from build123d import *

# Parameters (mm, degrees)
SKETCH1_W           = 297.73626
SKETCH1_H           = 182.7784
BOSS_EXTRUDE1_DEPTH = 15.24
CUT_EXTRUDE1_DEPTH  = 350.695698609
CUT_EXTRUDE2_DEPTH  = 350.695698609
SKETCH5_W           = 297.73626
SKETCH5_H           = 50.702926555
BOSS_EXTRUDE2_DEPTH = 76.2
FILLET1_R           = 12.7
FILLET2_R           = 12.7
SKETCH6_R           = 16.245750799
BOSS_EXTRUDE3_DEPTH = 50.8
SKETCH7_R           = 11.813796097
BOSS_EXTRUDE4_DEPTH = 12.7
CHAMFER1_SIZE       = 10
SKETCH8_R           = 1.248823532
CUT_EXTRUDE3_DEPTH  = 12.7
BOSS_EXTRUDE5_DEPTH = 12.7
BOSS_EXTRUDE6_DEPTH = 89.408
SKETCH11_W          = 104.0892
SKETCH11_H          = 178.532208179
BOSS_EXTRUDE7_DEPTH = 3.048
SKETCH12_R          = 15.475849778
SKETCH12_R_2        = 18.114114382
SKETCH12_R_3        = 14.983279797
BOSS_EXTRUDE8_DEPTH = 12.192


with BuildPart() as part:
    # Sketch1 → Boss-Extrude1 (new body)
    with BuildSketch(Plane(origin=(0, 0, 0), x_dir=(1, 0, 0), z_dir=(0, 1, 0))):
        with Locations((148.86813, 91.3892)):
            Rectangle(SKETCH1_W, SKETCH1_H)
    extrude(amount=BOSS_EXTRUDE1_DEPTH)

    # Sketch2 → Cut-Extrude1 (cut, through all)
    with BuildSketch(Plane.ZY):
        with BuildLine():
            ThreePointArc((-43.45432, 0), (-56.15432, 12.7), (-68.85432, 0))
            Line((-68.85432, 0), (-43.45432, 0))
        make_face()
        with BuildLine():
            ThreePointArc((-113.92408, 0), (-126.62408, 12.7), (-139.32408, 0))
            Line((-139.32408, 0), (-126.62408, 0))
            Line((-126.62408, 0), (-113.92408, 0))
        make_face()
    extrude(amount=-CUT_EXTRUDE1_DEPTH, mode=Mode.SUBTRACT)

    # Sketch4 → Cut-Extrude2 (cut, through all)
    with BuildSketch(Plane.ZY):
        with BuildLine():
            Line((-113.92408, 0), (-91.3892, 0))
            Line((-91.3892, 0), (-91.3892, 15.24))
            Line((-91.3892, 15.24), (-182.7784, 15.24))
            Line((-182.7784, 15.24), (-182.7784, 0))
            Line((-182.7784, 0), (-139.32408, 0))
            ThreePointArc((-139.32408, 0), (-126.62408, 12.7), (-113.92408, 0))
        make_face()
    extrude(amount=-CUT_EXTRUDE2_DEPTH, mode=Mode.SUBTRACT)

    # Sketch5 → Boss-Extrude2 (add)
    with BuildSketch(Plane(origin=(0, 15.24, 0), x_dir=(1, 0, 0), z_dir=(0, 1, 0))):
        with Locations((148.86813, 66.037736723)):
            Rectangle(SKETCH5_W, SKETCH5_H)
    extrude(amount=BOSS_EXTRUDE2_DEPTH)

    # Fillet1
    fillet1_edges = [part.edges().sort_by_distance(p)[0] for p in [
        (148.86813, 91.44, -91.3892),
    ]]
    fillet(fillet1_edges, radius=FILLET1_R)

    # Fillet2
    fillet2_edges = [part.edges().sort_by_distance(p)[0] for p in [
        (148.86813, 91.44, -40.686273445),
    ]]
    fillet(fillet2_edges, radius=FILLET2_R)

    # Sketch6 → Boss-Extrude3 (add)
    with BuildSketch(Plane.ZY):
        with Locations(Location((-66.037736722, 72.73477654, 0), (0, 0, 180))):
            Circle(SKETCH6_R)
    extrude(amount=BOSS_EXTRUDE3_DEPTH)

    # Sketch7 → Boss-Extrude4 (add)
    with BuildSketch(Plane.ZY.offset(50.8)):
        with Locations((-66.037736722, 72.73477654)):
            Circle(SKETCH7_R)
    extrude(amount=BOSS_EXTRUDE4_DEPTH)

    # Chamfer1
    chamfer1_edges = [part.edges().sort_by_distance(p)[0] for p in [
        (-63.5, 72.73477654, -77.851532819),
    ]]
    chamfer(chamfer1_edges, length=CHAMFER1_SIZE)

    # Sketch8 → Cut-Extrude3 (cut)
    with BuildSketch(Plane.ZY.offset(63.5)):
        with Locations((-66.037736722, 72.73477654)):
            Circle(SKETCH8_R)
    extrude(amount=-CUT_EXTRUDE3_DEPTH, mode=Mode.SUBTRACT)

    # Sketch9 → Boss-Extrude5 (add)
    with BuildSketch(Plane.XY):
        Polygon((297.73626, 0), (90.894406839, 0), (0, 67.007031279), (0, 91.44), (47.551027836, 178.532208179), (90.894406839, 178.532208179), (297.73626, 178.532208179), align=None)
        with BuildLine():
            Line((58.530996724, 73.070623488), (113.961199629, 73.070623488))
            ThreePointArc((113.961199629, 73.070623488), (119.349353302, 70.83877716), (121.581199629, 65.450623488))
            Line((121.581199629, 65.450623488), (121.581199629, 31.944306806))
            ThreePointArc((121.581199629, 31.944306806), (117.704665398, 25.307224312), (110.019293058, 25.423128034))
            Line((110.019293058, 25.423128034), (54.589090153, 58.929444715))
            ThreePointArc((54.589090153, 58.929444715), (51.190840655, 67.496719496), (58.530996724, 73.070623488))
        make_face(mode=Mode.SUBTRACT)
        with BuildLine():
            Line((265.539203866, 159.20856434), (166.955187388, 159.20856434))
            ThreePointArc((166.955187388, 159.20856434), (161.567033715, 156.976718013), (159.335187388, 151.58856434))
            Line((159.335187388, 151.58856434), (159.335187388, 110.936484564))
            ThreePointArc((159.335187388, 110.936484564), (161.567033715, 105.548330891), (166.955187388, 103.316484564))
            Line((166.955187388, 103.316484564), (265.539203866, 103.316484564))
            ThreePointArc((265.539203866, 103.316484564), (270.927357539, 105.548330891), (273.159203866, 110.936484564))
            Line((273.159203866, 110.936484564), (273.159203866, 151.58856434))
            ThreePointArc((273.159203866, 151.58856434), (270.927357539, 156.976718013), (265.539203866, 159.20856434))
        make_face(mode=Mode.SUBTRACT)
        with BuildLine():
            Line((144.177739207, 65.450623488), (144.177739207, 46.629358654))
            ThreePointArc((144.177739207, 46.629358654), (148.790363397, 39.627923749), (157.043904755, 41.102863649))
            Line((157.043904755, 41.102863649), (176.87088603, 59.924128483))
            ThreePointArc((176.87088603, 59.924128483), (178.70201841, 68.274849759), (171.624720482, 73.070623488))
            Line((171.624720482, 73.070623488), (151.797739207, 73.070623488))
            ThreePointArc((151.797739207, 73.070623488), (146.409585534, 70.83877716), (144.177739207, 65.450623488))
        make_face(mode=Mode.SUBTRACT)
        with BuildLine():
            Line((183.099865501, 18.43421436), (163.272884226, 18.43421436))
            ThreePointArc((163.272884226, 18.43421436), (156.195586298, 23.229988089), (158.026718678, 31.580709365))
            Line((158.026718678, 31.580709365), (177.853699953, 50.401974198))
            ThreePointArc((177.853699953, 50.401974198), (186.107241311, 51.876914099), (190.719865501, 44.875479193))
            Line((190.719865501, 44.875479193), (190.719865501, 26.05421436))
            ThreePointArc((190.719865501, 26.05421436), (188.488019173, 20.666060687), (183.099865501, 18.43421436))
        make_face(mode=Mode.SUBTRACT)
        with BuildLine():
            Line((215.002714002, 65.450623488), (215.002714002, 45.672508012))
            ThreePointArc((215.002714002, 45.672508012), (219.472522634, 38.734158472), (227.638066848, 39.935728791))
            Line((227.638066848, 39.935728791), (250.261137525, 59.713844266))
            ThreePointArc((250.261137525, 59.713844266), (252.379460368, 68.129255819), (245.245784679, 73.070623488))
            Line((245.245784679, 73.070623488), (222.622714002, 73.070623488))
            ThreePointArc((222.622714002, 73.070623488), (217.234560329, 70.83877716), (215.002714002, 65.450623488))
        make_face(mode=Mode.SUBTRACT)
        with BuildLine():
            Line((235.296133189, 18.43421436), (257.919203866, 18.43421436))
            ThreePointArc((257.919203866, 18.43421436), (263.307357539, 20.666060687), (265.539203866, 26.05421436))
            Line((265.539203866, 26.05421436), (265.539203866, 45.832329836))
            ThreePointArc((265.539203866, 45.832329836), (261.069395235, 52.770679376), (252.903851021, 51.569109057))
            Line((252.903851021, 51.569109057), (230.280780343, 31.790993581))
            ThreePointArc((230.280780343, 31.790993581), (228.1624575, 23.375582029), (235.296133189, 18.43421436))
        make_face(mode=Mode.SUBTRACT)
    extrude(amount=BOSS_EXTRUDE5_DEPTH)

    # Sketch10 → Boss-Extrude6 (add)
    with BuildSketch(Plane(origin=(0, 0, 0), x_dir=(-1, 0, 0), z_dir=(0, 0, -1))):
        Polygon((-47.58427569, 178.532208179), (0, 91.44), (-8.220392821, 91.44), (-52.613193371, 172.690937859), (-297.73626, 172.690937859), (-297.73626, 178.532208179), align=None)
    extrude(amount=BOSS_EXTRUDE6_DEPTH)

    # Sketch11 → Boss-Extrude7 (add)
    with BuildSketch(Plane(origin=(297.73626, 0, 0), x_dir=(0, 0, -1), z_dir=(1, 0, 0))):
        with Locations((39.3446, 89.26610409)):
            Rectangle(SKETCH11_W, SKETCH11_H)
    extrude(amount=BOSS_EXTRUDE7_DEPTH)

    # Sketch12 → Boss-Extrude8 (add)
    with BuildSketch(Plane(origin=(300.78426, 0, 0), x_dir=(0, 0, -1), z_dir=(1, 0, 0))):
        with Locations(Location((57.905976466, 26.649412399, 0), (0, 0, 180))):
            Circle(SKETCH12_R)
        with Locations(Location((42.430126688, 89.26610409, 0), (0, 0, 180))):
            Circle(SKETCH12_R_2)
        with Locations(Location((14.521554365, 26.649412399, 0), (0, 0, 180))):
            Circle(SKETCH12_R_3)
    extrude(amount=BOSS_EXTRUDE8_DEPTH)


solid = part.part
Model file for the job. Use its own axes, mm. A direction names the side the tool comes from. Round coordinates to 2 decimals unless told otherwise and drop trailing zeros. Loops run counter-clockwise (first coordinate to the right, second up) from the corner with the lowest first, then second, coordinate; pieces in that order, holes last. Notation, with made-up numbers: (85, -8) -> (128, -8) arc R14 ccw to (128, 12) -> close; hole circle Ø1 at (39.25, 25.5). An arc over 180 degrees is marked (long way). Answer as CSV lines item,"result". Start each with the question number.
1) Pin check, flat tips, straight feed: P1, Ø10, axis at x = 249.5, y = 109, coming from the -Z side; P2, Ø4, axis at y = 146.5, z = -57, coming from the -X side; P3, Ø2, axis at y = 144.5, z = -78, coming from the +X side; P4, Ø6.5, axis at y = 4, z = -60.5, coming from the -X side. Stop position of each tip, or through.
2) Slice it at B-B (z = -37). List the corners of the cut face in (x, y), plus the area to 3 significant figures.
3) Slice it at C-C (z = -15). List the corners of the cut face in (x, y).
4) Tool access for faces 1 (the face through (-52.13, 73.25, -77.84)), 2 (the face through (217, 159.209, 6)), 3 (the face through (151, 95, 0)): list every direction of +Z, -Z, +X, -X, +Y, -Y with a clear straight run to the whole face (end or side of a thin tool).
5) Slice it at A-A (x = 187). List the corners of the cut face in (y, z), plus the area to 3 significant figures.
6) Mould opens along X. For faces 4 (the face through (300.784, 110, -39)), 5 (the face through (148, 88, 12.7)), 6 (the face through (166.819, 50.382, 6.261)) say: +X half, -X half, draft (parallel to the pull), parting line (faces both ways), or undercut.
7) Probe line 1 along Z through (x, y) = (292, 48); line 2 along Y through (x, z) = (100.5, -10); line 3 along Z through (x, y) = (110, 153). List the from-to ranges inside material, lowest first.
Filled in:
1,P1,"passes through"
1,P2,"stops at x = 28.99"
1,P3,"stops at x = 300.78"
1,P4,"stops at x = 297.74"
2,outline,"(0, 0) -> (300.78, 0) -> (300.78, 71.99) -> (312.98, 71.99) -> (312.98, 106.55) -> (300.78, 106.55) -> (300.78, 178.53) -> (47.58, 178.53) -> (0, 91.44) -> (8.22, 91.44) -> (52.61, 172.69) -> (297.74, 172.69) -> (297.74, 15.24) -> (0, 15.24) -> close"
2,area,"7,640 mm2"
3,outline,"(0, 0) -> (300.78, 0) -> (300.78, 11.67) -> (312.98, 11.67) -> (312.98, 41.63) -> (300.78, 41.63) -> (300.78, 178.53) -> (47.58, 178.53) -> (0, 91.44) -> (8.22, 91.44) -> (52.61, 172.69) -> (297.74, 172.69) -> (297.74, 15.24) -> (0, 15.24) -> close"
4,face 1,"-X"
4,face 2,"+Z, -Z"
4,face 3,"none"
5,outline,"(0, -91.39) -> (78.74, -91.39) arc R12.7 ccw to (91.44, -78.69) -> (91.44, -53.39) arc R12.7 ccw to (78.74, -40.69) -> (15.24, -40.69) -> (15.24, 0) -> (19.51, 0) -> (19.51, 12.7) -> (0, 12.7) -> (0, -43.45) arc R12.7 cw to (0, -68.85) -> close; (51.42, 0) -> (103.32, 0) -> (103.32, 12.7) -> (51.42, 12.7) -> close; (159.21, 0) -> (172.69, 0) -> (172.69, -89.41) -> (178.53, -89.41) -> (178.53, 12.7) -> (159.21, 12.7) -> close"
5,area,"6,610 mm2"
6,face 4,"+X half"
6,face 5,"draft"
6,face 6,"undercut"
7,line 1,"z = -91.39 to -40.69, 0 to 12.7"
7,line 2,"y = 0 to 15.24, 172.69 to 178.53"
7,line 3,"z = 0 to 12.7"
